Autodesk Inventor part; units mm, degrees
ref_plane "YZ Plane" through (0, 0, 0) normal (1, 0, 0) x (0, 1, 0)
ref_plane "XZ Plane" through (0, 0, 0) normal (0, 1, 0) x (-1, 0, 0)
ref_plane "XY Plane" through (0, 0, 0) normal (0, 0, 1) x (1, 0, 0)
sketch "Sketch1" plane through (0, 0, 0) normal (0, 0, 1) x (1, 0, 0)
  circle A0 centre (0, 0) radius 11.5
  circle A1 centre (0, 0) radius 25
  line L0 (-1.315, 13.9381) -> (-1.315, 23.3542)
  line L1 (-1.315, 23.3542) -> (-4.9641, 23.3542)
  line L2 (-4.9641, 23.3542) -> (-5.1978, 24.4537)
  line L3 (1.315, 13.9381) -> (1.315, 23.3542)
  line L4 (1.315, 23.3542) -> (4.9641, 23.3542)
  line L5 (4.9641, 23.3542) -> (5.1978, 24.4537)
  arc A2 (5.1978, 24.4537) -> (-5.1978, 24.4537) centre (0, 0) ccw
  circle A3 centre (0, 0) radius 14
  line L6 (-8.1079, 11.4133) -> (-12.8159, 19.5679)
  line L7 (-12.8159, 19.5679) -> (-15.9762, 17.7433)
  line L8 (-15.9762, 17.7433) -> (-16.7283, 18.5786)
  line L9 (-5.8303, 12.7282) -> (-10.5383, 20.8829)
  line L10 (-10.5383, 20.8829) -> (-7.3781, 22.7074)
  line L11 (-7.3781, 22.7074) -> (-7.7254, 23.7764)
  arc A4 (-7.7254, 23.7764) -> (-16.7283, 18.5786) centre (0, 0) ccw
  line L12 (-12.7282, 5.8303) -> (-20.8829, 10.5383)
  line L13 (-20.8829, 10.5383) -> (-22.7074, 7.3781)
  line L14 (-22.7074, 7.3781) -> (-23.7764, 7.7254)
  line L15 (-11.4133, 8.1079) -> (-19.5679, 12.8159)
  line L16 (-19.5679, 12.8159) -> (-17.7433, 15.9762)
  line L17 (-17.7433, 15.9762) -> (-18.5786, 16.7283)
  arc A5 (-18.5786, 16.7283) -> (-23.7764, 7.7254) centre (0, 0) ccw
  line L18 (-13.9381, -1.315) -> (-23.3542, -1.315)
  line L19 (-23.3542, -1.315) -> (-23.3542, -4.9641)
  line L20 (-23.3542, -4.9641) -> (-24.4537, -5.1978)
  line L21 (-13.9381, 1.315) -> (-23.3542, 1.315)
  line L22 (-23.3542, 1.315) -> (-23.3542, 4.9641)
  line L23 (-23.3542, 4.9641) -> (-24.4537, 5.1978)
  arc A6 (-24.4537, 5.1978) -> (-24.4537, -5.1978) centre (0, 0) ccw
  line L24 (-11.4133, -8.1079) -> (-19.5679, -12.8159)
  line L25 (-19.5679, -12.8159) -> (-17.7433, -15.9762)
  line L26 (-17.7433, -15.9762) -> (-18.5786, -16.7283)
  line L27 (-12.7282, -5.8303) -> (-20.8829, -10.5383)
  line L28 (-20.8829, -10.5383) -> (-22.7074, -7.3781)
  line L29 (-22.7074, -7.3781) -> (-23.7764, -7.7254)
  arc A7 (-23.7764, -7.7254) -> (-18.5786, -16.7283) centre (0, 0) ccw
  line L30 (-5.8303, -12.7282) -> (-10.5383, -20.8829)
  line L31 (-10.5383, -20.8829) -> (-7.3781, -22.7074)
  line L32 (-7.3781, -22.7074) -> (-7.7254, -23.7764)
  line L33 (-8.1079, -11.4133) -> (-12.8159, -19.5679)
  line L34 (-12.8159, -19.5679) -> (-15.9762, -17.7433)
  line L35 (-15.9762, -17.7433) -> (-16.7283, -18.5786)
  arc A8 (-16.7283, -18.5786) -> (-7.7254, -23.7764) centre (0, 0) ccw
  line L36 (1.315, -13.9381) -> (1.315, -23.3542)
  line L37 (1.315, -23.3542) -> (4.9641, -23.3542)
  line L38 (4.9641, -23.3542) -> (5.1978, -24.4537)
  line L39 (-1.315, -13.9381) -> (-1.315, -23.3542)
  line L40 (-1.315, -23.3542) -> (-4.9641, -23.3542)
  line L41 (-4.9641, -23.3542) -> (-5.1978, -24.4537)
  arc A9 (-5.1978, -24.4537) -> (5.1978, -24.4537) centre (0, 0) ccw
  line L42 (8.1079, -11.4133) -> (12.8159, -19.5679)
  line L43 (12.8159, -19.5679) -> (15.9762, -17.7433)
  line L44 (15.9762, -17.7433) -> (16.7283, -18.5786)
  line L45 (5.8303, -12.7282) -> (10.5383, -20.8829)
  line L46 (10.5383, -20.8829) -> (7.3781, -22.7074)
  line L47 (7.3781, -22.7074) -> (7.7254, -23.7764)
  arc A10 (7.7254, -23.7764) -> (16.7283, -18.5786) centre (0, 0) ccw
  line L48 (12.7282, -5.8303) -> (20.8829, -10.5383)
  line L49 (20.8829, -10.5383) -> (22.7074, -7.3781)
  line L50 (22.7074, -7.3781) -> (23.7764, -7.7254)
  line L51 (11.4133, -8.1079) -> (19.5679, -12.8159)
  line L52 (19.5679, -12.8159) -> (17.7433, -15.9762)
  line L53 (17.7433, -15.9762) -> (18.5786, -16.7283)
  arc A11 (18.5786, -16.7283) -> (23.7764, -7.7254) centre (0, 0) ccw
  line L54 (13.9381, 1.315) -> (23.3542, 1.315)
  line L55 (23.3542, 1.315) -> (23.3542, 4.9641)
  line L56 (23.3542, 4.9641) -> (24.4537, 5.1978)
  line L57 (13.9381, -1.315) -> (23.3542, -1.315)
  line L58 (23.3542, -1.315) -> (23.3542, -4.9641)
  line L59 (23.3542, -4.9641) -> (24.4537, -5.1978)
  arc A12 (24.4537, -5.1978) -> (24.4537, 5.1978) centre (0, 0) ccw
  line L60 (11.4133, 8.1079) -> (19.5679, 12.8159)
  line L61 (19.5679, 12.8159) -> (17.7433, 15.9762)
  line L62 (17.7433, 15.9762) -> (18.5786, 16.7283)
  line L63 (12.7282, 5.8303) -> (20.8829, 10.5383)
  line L64 (20.8829, 10.5383) -> (22.7074, 7.3781)
  line L65 (22.7074, 7.3781) -> (23.7764, 7.7254)
  arc A13 (23.7764, 7.7254) -> (18.5786, 16.7283) centre (0, 0) ccw
  line L66 (5.8303, 12.7282) -> (10.5383, 20.8829)
  line L67 (10.5383, 20.8829) -> (7.3781, 22.7074)
  line L68 (7.3781, 22.7074) -> (7.7254, 23.7764)
  line L69 (8.1079, 11.4133) -> (12.8159, 19.5679)
  line L70 (12.8159, 19.5679) -> (15.9762, 17.7433)
  line L71 (15.9762, 17.7433) -> (16.7283, 18.5786)
  arc A14 (16.7283, 18.5786) -> (7.7254, 23.7764) centre (0, 0) ccw
  dimension "d1" = 50
  dimension "d0" = 23
  dimension "d2" = 24
  dimension "d3" = 28
  dimension "d6" = 360
extrude "Extrusion1" add sketch "Sketch1" along normal blind 30 contours A3 | L5 L4 L3 A3 L0 L1 L2 A1
pattern_circular "Circular Pattern1" count 12 over 360 about axis through (0, 0, -10) along (0, 0, 1) of "Extrusion1"
equation "\"d1\" = stator_diameter"
equation "\"d0\" = stator_id"
equation "\"d8\" = stator_length"
equation "\"stator_length\" = 30"
equation "\"stator_id\" = 23"
properties part number "Stator" material "Steel, Mild, Welded"
Verification items for the finished model (mm, model axes). A direction names the side the tool comes from. Give positions to 0.01 mm unless a question says otherwise; leave off trailing zeros. Order: outer loops, then holes, each group sorted by start corner. A loop starts at its lowest first (then second) coordinate and runs counter-clockwise, first axis right, second up. Notation, with made-up numbers: (27.5, -10) - (32.5, -10) arc R27 cw to (32.5, 23) - close; hole circle Ø6 at (45.25, 31.25). An arc over 180 degrees is marked (long way). Answer as CSV lines item,"result". Start each with the question number.
Item 1: Mould release check, pull along Y, two halves, no side actions. Record for faces 3 (the face through (-25, 0, 15)), 4 (the face through (3, 23.354, 15)), 5 (the face through (14.37, 18.67, 14.79)), 6 (the face through (-21.614, -12.563, 14.79)): released by +Y, released by -Y, zero draft, split by the parting line, or undercut.
Item 2: Material ranges on L1, parallel to X at y = 10, z = 27.25; L2, parallel to X at y = -19, z = 14.5 (3 decimals); L3, parallel to Y at x = -21.5, z = 28.75 (3 decimals), recorded low to high.
Item 3: Section check C-C, the plane y = 15. Record the boundary of the cut face in (x, z) (3 decimals).
Item 4: Gauge pin test, flat ends, axial feed: pin 1 (1.8 mm diameter, centred on x = -3.5, z = 8.5, fed in from +Y); pin 2 (1.8 mm diameter, centred on x = -3.5, z = 14, fed in from -Y); pin 3 (2 mm diameter, centred on x = 12, z = 7, fed in from -Y); pin 4 (18.5 mm diameter, centred on x = 0, y = 0, fed in from -Z). Record the tip position at first contact, or that the pin passes through.
Item 5: Section check A-A, the plane x = 0. Record the boundary of the cut face in (y, z).
Item 6: Access from +Z, -Z, +X, -X, +Y, -Y to the whole of each face (thin tool, end or side, straight path). Record for faces 1 (the face through (8.15, -16.75, 14.79)), 2 (the face through (0, -25, 15)).
Filled in:
1,face 3,"split by the parting line"
1,face 4,"undercut"
1,face 5,"undercut"
1,face 6,"released by -Y"
2,L1,"-22.91 to -21.19, -19.95 to -14.69, -9.8 to -5.68, 5.68 to 9.8, 14.69 to 19.95, 21.19 to 22.91"
2,L2,"-16.248 to -13.799, -12.488 to -9.451, -1.315 to 1.315, 9.451 to 12.488, 13.799 to 16.248"
2,L3,"-12.757 to -9.469, -1.315 to 1.315, 9.469 to 12.757"
3,outline,"(-20, 0) - (-18.307, 0) - (-18.307, 30) - (-20, 30) - close; (-10.179, 0) - (-7.142, 0) - (-7.142, 30) - (-10.179, 30) - close; (-1.315, 0) - (1.315, 0) - (1.315, 30) - (-1.315, 30) - close; (7.142, 0) - (10.179, 0) - (10.179, 30) - (7.142, 30) - close; (18.307, 0) - (20, 0) - (20, 30) - (18.307, 30) - close"
4,pin 1,"y = 24.86"
4,pin 2,"y = -24.86"
4,pin 3,"y = -22.45"
4,pin 4,"through"
5,outline,"(-25, 0) - (-11.5, 0) - (-11.5, 30) - (-25, 30) - close; (11.5, 0) - (25, 0) - (25, 30) - (11.5, 30) - close"
6,face 1,"+Z, -Z"
6,face 2,"+Z, -Z, -Y"
